Part model, mm, in its own coordinate system. Round coordinates to 2 decimals unless told otherwise and drop trailing zeros. Write each loop counter-clockwise with the first axis right and the second up, starting at its lowest first coordinate (ties: lowest second). Pieces come first, ordered by that corner, then holes. Notation, with made-up numbers: M 36.25,-1.75 L 89.25,-1.75 A32 ccw 89.25,37.25 Z; hole C 45.25,9.25 d6. An arc over 180 degrees is marked long. Answer as a JSON object with one key per item and string values. Group by question number.
1. Band-saw the part on B-B, the plane z = -0.15. Write the cut outline in (x, y), plus the area to 3 significant figures.
2. Band-saw the part on C-C, the plane x = 9. Write the cut outline in (y, z).
3. Band-saw the part on A-A, the plane x = 14. Write the cut outline in (y, z), plus the area to 3 significant figures.
4. Band-saw the part on D-D, the plane y = 5. Count the separate pieces of the cut face and the enclosed holes in it, plus the area to 3 significant figures.
5. Drill centre lines: line 1 (X direction, y = 5, z = 0.05); line 2 (Y direction, x = -14, z = -0.1); line 3 (Z direction, x = 9, y = 13). Where is each one in solid material? Low to high. Write a range as from..to.
from build123d import *

# Parameters (mm, degrees)
SKETCH1_W           = 35
SKETCH1_H           = 2
BOSS_EXTRUDE1_DEPTH = 14
SKETCH2_R           = 1.75
CUT_EXTRUDE1_DEPTH  = 14
SKETCH3_R           = 0.5
CUT_EXTRUDE2_DEPTH  = 23.433234274
LPATTERN1_COUNT     = 18
LPATTERN1_PITCH     = 2
FILLET1_R           = 0.15


with BuildPart() as part:
    # Sketch1 → Boss-Extrude1 (new body)
    with BuildSketch(Plane(origin=(0, 0, 0), x_dir=(1, 0, 0), z_dir=(0, 1, 0))):
        Rectangle(SKETCH1_W, SKETCH1_H)
    extrude(amount=BOSS_EXTRUDE1_DEPTH)

    # Sketch2 → Cut-Extrude1 (cut)
    with BuildSketch(Plane.XY.offset(1)):
        with Locations((-14, 5)):
            Circle(SKETCH2_R)
        with Locations((14, 5)):
            Circle(SKETCH2_R)
    extrude(amount=-CUT_EXTRUDE1_DEPTH, mode=Mode.SUBTRACT)

    # Sketch3 → Cut-Extrude2 (cut, through all)
    with BuildSketch(Plane(origin=(0, 14, 0), x_dir=(1, 0, 0), z_dir=(0, 1, 0))):
        with Locations((-17, -1)):
            Circle(SKETCH3_R)
    cut_extrude2 = extrude(amount=-CUT_EXTRUDE2_DEPTH, mode=Mode.SUBTRACT)

    # LPattern1: Cut-Extrude2 ×18
    with Locations(*[(i * LPATTERN1_PITCH, 0, 0) for i in range(1, LPATTERN1_COUNT)]):
        add(cut_extrude2, mode=Mode.SUBTRACT)

    # Fillet1
    fillet1_edges = [part.edges().sort_by_distance(p)[0] for p in [
        (-16.5, 7, 1),
        (-17.5, 7, 1),
        (-14.5, 10.338525492, 1),
        (-15.5, 9.950693909, 1),
        (13.5, 1.661474508, 1),
        (12.5, 2.049306091, 1),
        (15.5, 2.049306091, 1),
        (14.5, 1.661474508, 1),
        (17.5, 7, 1),
        (16.5, 7, 1),
        (15.5, 9.950693909, 1),
        (14.5, 10.338525492, 1),
        (13.5, 10.338525492, 1),
        (12.5, 9.950693909, 1),
        (11.5, 7, 1),
        (10.5, 7, 1),
        (9.5, 7, 1),
        (8.5, 7, 1),
        (7.5, 7, 1),
        (6.5, 7, 1),
        (5.5, 7, 1),
        (4.5, 7, 1),
        (3.5, 7, 1),
        (2.5, 7, 1),
        (1.5, 7, 1),
        (0.5, 7, 1),
        (-0.5, 7, 1),
        (-1.5, 7, 1),
        (-2.5, 7, 1),
        (-3.5, 7, 1),
        (-4.5, 7, 1),
        (-5.5, 7, 1),
        (-6.5, 7, 1),
        (-7.5, 7, 1),
        (-8.5, 7, 1),
        (-9.5, 7, 1),
        (-12.5, 9.950693909, 1),
        (-13.5, 10.338525492, 1),
        (-10.5, 7, 1),
        (-11.5, 7, 1),
        (-12.5, 2.049306091, 1),
        (-13.5, 1.661474508, 1),
        (-14.5, 1.661474508, 1),
        (-15.5, 2.049306091, 1),
    ]]
    fillet(fillet1_edges, radius=FILLET1_R)


solid = part.part
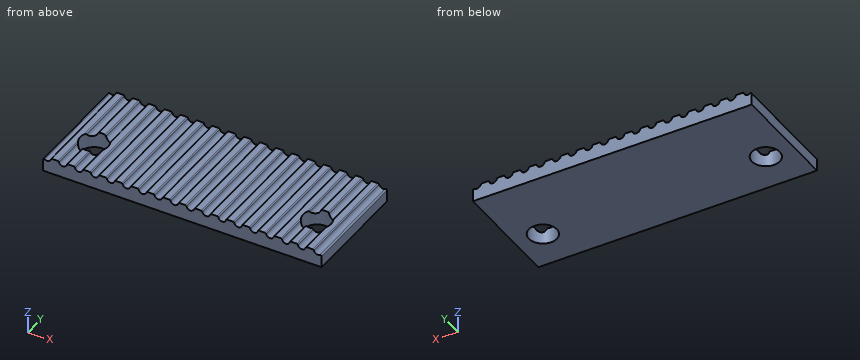
Worked answers:
{
 "1": {"outline": "M -17.5,0 L 17.5,0 L 17.5,14 L -17.5,14 Z; hole C -14,5 d3.5; hole C 14,5 d3.5", "area": "471 mm^2"},
 "2": {"outline": "M 0,-1 L 14,-1 L 14,0.5 L 0,0.5 Z"},
 "3": {"outline": "M 0,-1 L 3.25,-1 L 3.25,1 L 0,1 Z; M 6.75,-1 L 14,-1 L 14,1 L 6.75,1 Z", "area": "21.0 mm^2"},
 "4": {"separate pieces": "3", "enclosed holes": "0", "area": "50.4 mm^2"},
 "5": {"line 1": "x = -17.5..-15.75, -12.25..12.25, 15.75..17.5", "line 2": "y = 0..3.25, 6.75..14", "line 3": "z = -1..0.5"}
}
